Geometry: final body of the model. Coordinates: model frame, mm. Face numbers are marked on the shaded views. A direction names the side the tool comes from. Give positions to 0.01 mm unless a question says otherwise; leave off trailing zeros. Order: outer loops, then holes, each group sorted by start corner. A loop starts at its lowest first (then second) coordinate and runs counter-clockwise, first axis right, second up. Notation, with made-up numbers: M -3,41 L 34,41 A18 cw 34,45 Z; hole C -6,34 d9. An arc over 180 degrees is marked long. One line per item, written item: value. Start each with the question number.
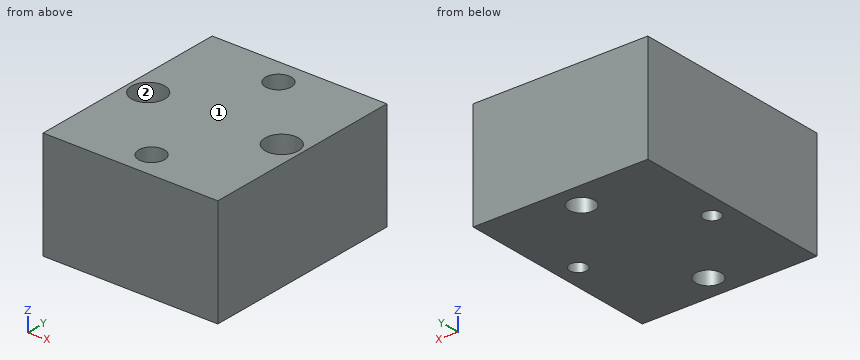
```python
from build123d import *

# Parameters (mm, degrees)
F0_W           = 34
F0_H           = 40
F1_DEPTH       = 21
F3_D           = 3.3
F3_CBORE_D     = 6.5
F3_CBORE_DEPTH = 10
F4_D           = 5


with BuildPart() as f1:
    # F0 (on Top) → F1 (new body)
    with BuildSketch(Plane.XY):
        with Locations((-19.8004702032, -43.8329163194)):
            Rectangle(F0_W, F0_H)
    extrude(amount=F1_DEPTH)

    # F3 (through all)
    with Locations(Plane.XY.offset(21)):
        with Locations((-32.8004702032, -43.8329163194), (-6.8004702032, -43.8329163194)):
            CounterBoreHole(F3_D / 2, F3_CBORE_D / 2, F3_CBORE_DEPTH)

    # F4 (through all)
    with Locations(Plane.XY.offset(21)):
        with Locations((-19.8004702032, -28.8329163194), (-19.8004702032, -58.8329163194)):
            Hole(F4_D / 2)


solid = f1.part
```
Q1. Section query B-B on z = 6. Return loops of the section in (x, y).
Q2. Section query A-A on x = -20.5. Return loops of the section in (y, z).
Q3. Contact query for flat-ended pins moving along their axis: pin 1 (3 mm diameter, centred on x = -6.5, y = -42.5, fed in from +Z); pin 2 (3 mm diameter, centred on x = -6.8, y = -43.83, fed in from -Z). Output: stop coordinate, or through.
Q4. Ray query, line 1 along Y through (x, z) = (-7, 16.25); line 2 along Y through (x, z) = (-20, 19); line 3 along X through (y, z) = (-42, 13). Return the intervals inside material, ascending. Write a range as [from, to].
Q5. Set-up query: the marked faces 1 and 2. Return all of +Z, -Z, +X, -X, +Y, -Y with unobstructed straight access to the full face (end or side cutting, diameter ignored); none if empty.
Q6. Section query C-C on x = -7.5. Return loops of the section in (y, z).
Q7. Section query D-D on z = 11.5. Return loops of the section in (x, y), and give its area (3 significant figures).
Results below:
1. outline: M -36.8,-63.83 L -2.8,-63.83 L -2.8,-23.83 L -36.8,-23.83 Z; hole C -32.8,-43.83 d3.3; hole C -19.8,-58.83 d5; hole C -19.8,-28.83 d5; hole C -6.8,-43.83 d3.3
2. outline: M -63.83,0 L -61.23,0 L -61.23,21 L -63.83,21 Z; M -56.43,0 L -31.23,0 L -31.23,21 L -56.43,21 Z; M -26.43,0 L -23.83,0 L -23.83,21 L -26.43,21 Z
3. pin 1: z = 11
3. pin 2: through
4. line 1: [-63.83, -47.08], [-40.59, -23.83]
4. line 2: [-63.83, -61.32], [-56.34, -31.32], [-26.34, -23.83]
4. line 3: [-36.8, -35.48], [-30.12, -9.48], [-4.12, -2.8]
5. face 1: +Z, +X, -X, +Y, -Y
5. face 2: +Z
6. outline: M -63.83,0 L -45.33,0 L -45.33,11 L -47.01,11 L -47.01,21 L -63.83,21 Z; M -42.34,0 L -23.83,0 L -23.83,21 L -40.66,21 L -40.66,11 L -42.34,11 Z
7. outline: M -36.8,-63.83 L -2.8,-63.83 L -2.8,-23.83 L -36.8,-23.83 Z; hole C -32.8,-43.83 d6.5; hole C -19.8,-58.83 d5; hole C -19.8,-28.83 d5; hole C -6.8,-43.83 d6.5
7. area: 1,250 mm2
